Autodesk Fusion 360 part; units mm, degrees
sketch "Sketch1" plane through (0, 0, 0) normal (0, 0, 1) x (1, 0, 0)
  circle A0 centre (0, 0) radius 2.5
  line L0 (0.2796, 2.4843) -> (10.2796, 19.8048)
  line L1 (10.2796, 19.8048) -> (12.0117, 18.8048)
  line L2 (12.0117, 18.8048) -> (2.0117, 1.4843)
  line L3 (-0.2796, 2.4843) -> (-10.2796, 19.8048)
  line L4 (-10.2796, 19.8048) -> (-12.0117, 18.8048)
  line L5 (-12.0117, 18.8048) -> (-2.0117, 1.4843)
  line L6 (-2.0117, -1.4843) -> (-12.0117, -18.8048)
  line L7 (-12.0117, -18.8048) -> (-10.2796, -19.8048)
  line L8 (-10.2796, -19.8048) -> (-0.2796, -2.4843)
  line L9 (2.0117, -1.4843) -> (12.0117, -18.8048)
  line L10 (12.0117, -18.8048) -> (10.2796, -19.8048)
  line L11 (10.2796, -19.8048) -> (0.2796, -2.4843)
  line L12 (20, 0) -> (16, 0)
  dimension "d1" = 5
  dimension "d3" = 2
  dimension "d4" = 20
  dimension "d6" = 2
  dimension "d7" = 20
  dimension "d8" = 20
  dimension "d9" = 20
  dimension "d11" = 2
  dimension "d12" = 20
  dimension "d13" = 20
  dimension "d14" = 2
  dimension "d16" = 20
  dimension "d17" = 20
  dimension "d18" = 120
  dimension "d19" = 120
  dimension "d20" = 60
  dimension "d21" = 60
extrude "Extrude1" add sketch "Sketch1" along normal blind 1 contours A0 L0 L1 L2 | A0 L9 L10 L11 | A0 L3 L4 L5 | A0 L6 L7 L8 makes body 1 at (7.8471, 13.5916, 0) makes body 2 at (7.8471, -13.5916, 0) makes body 3 at (-7.8471, 13.5916, 0) makes body 4 at (-7.8471, -13.5916, 0)
extrude "Extrude2" add sketch "Sketch1" along normal blind 18 contours A0 bodies 1 2 3 4
sketch "Sketch2" plane through (0, 0, 18) normal (0, 0, 1) x (-1, 0, 0)
  circle A0 centre (0, 0) radius 2.5
  line L0 (-2, -4) -> (-1, -4)
  line L1 (-1, -4) -> (-1, 4)
  line L2 (-1, 4) -> (-2, 4)
  line L3 (-2, 4) -> (-2, -4)
  line L4 (2, -4) -> (1, -4)
  line L5 (1, -4) -> (1, 4)
  line L6 (1, 4) -> (2, 4)
  line L7 (2, 4) -> (2, -4)
  line L8 (-2, -3) -> (-1, -3)
  line L9 (-2, 3) -> (-1, 3)
  line L10 (1, -3) -> (2, -3)
  line L11 (1, 3) -> (2, 3)
  dimension "d26" = 8
  dimension "d27" = 8
  dimension "d30" = 1
  dimension "d31" = 1
  dimension "d32" = 2
  dimension "d33" = 4
  dimension "d34" = 1
  dimension "d35" = 1
  dimension "d36" = 1
  dimension "d37" = 1
  dimension "d40" = 1
extrude "Extrude3" add sketch "Sketch2" along normal blind 1 contours A0 L5 L7 | A0 L5 L7 L11 | A0 L5 L7 L10 | A0 L1 L3 | A0 L1 L3 L9 | A0 L1 L3 L8 bodies 1
extrude "Extrude4" add sketch "Sketch2" along normal blind 15 contours L5 L6 L7 L11 | L4 L5 L7 L10 | L1 L2 L3 L9 | L0 L1 L3 L8 bodies 1
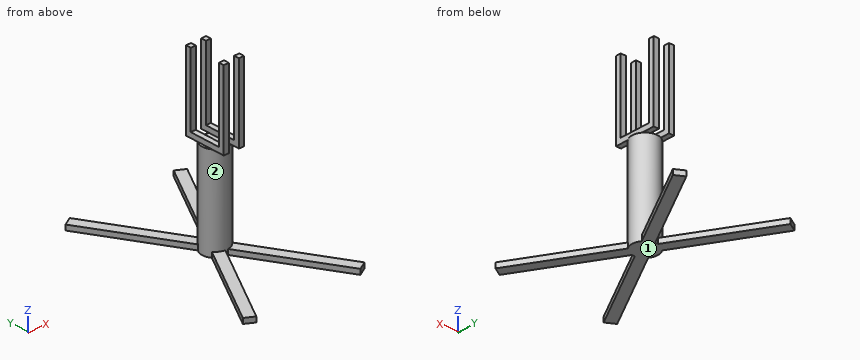
Verification items for the finished model (mm, model axes). Face numbers are marked on the shaded views. Round coordinates to 2 decimals unless told otherwise and drop trailing zeros. Order: outer loops, then holes, each group sorted by start corner. A loop starts at its lowest first (then second) coordinate and runs counter-clockwise, first axis right, second up.
1) Cross-section at C-C, the plane x = -4. Record the cut outline in (y, z), plus the area to 3 significant figures.
Geometry says:
outline: (-8.93, 0) - (-4.93, 0) - (-4.93, 1) - (-8.93, 1) - close; (4.93, 0) - (8.93, 0) - (8.93, 1) - (4.93, 1) - close
area: 8.00 mm2
2) Cross-section at A-A, the plane z = 19.5. Record the cut outline in (x, y).
Geometry says:
outline: (-2, -4) - (-1, -4) - (-1, -3) - (-2, -3) - close; (-2, 3) - (-1, 3) - (-1, 4) - (-2, 4) - close; (1, -4) - (2, -4) - (2, -3) - (1, -3) - close; (1, 3) - (2, 3) - (2, 4) - (1, 4) - close
3) Material ranges on line 1 (Z direction, x = 3.25, y = 6), recorded low to high.
Geometry says:
line 1: z = 0 to 1
4) Cross-section at D-D, the plane y = -16. Record the cut outline in (x, z).
Geometry says:
outline: (-10.39, 0) - (-8.08, 0) - (-8.08, 1) - (-10.39, 1) - close; (8.08, 0) - (10.39, 0) - (10.39, 1) - (8.08, 1) - close
5) Depth check by flat-ended pin: pin 1 (0.8 mm diameter, centred on x = -1.5, y = -3, fed in from -Z); pin 2 (4 mm diameter, centred on x = 5.5, z = 9.5, fed in from +Y); pin 3 (6.5 mm diameter, centred on y = 2, z = 27.5, fed in from +X); pin 4 (0.5 mm diameter, centred on x = 1.5, z = 26.5, fed in from -Y). Enter the tip coordinate at first touch or a pass-through.
Geometry says:
pin 1: stops at z = 0
pin 2: passes through
pin 3: stops at x = 2
pin 4: stops at y = -4
6) Draft check along Z on the marked faces 1 and 2. Enter one of: +Z half, -Z half, draft (parallel to the pull), parting line (faces both ways), or undercut.
Geometry says:
face 1: -Z half
face 2: undercut
7) Cross-section at B-B, the plane y = 0. Record the cut outline in (x, z).
Geometry says:
outline: (-2.5, 0) - (2.5, 0) - (2.5, 18) - (2, 18) - (2, 19) - (1, 19) - (1, 18) - (-1, 18) - (-1, 19) - (-2, 19) - (-2, 18) - (-2.5, 18) - close
